Autodesk Inventor part; units mm, degrees
ref_plane "Work Plane1" through (-20, 3, 0) normal (0, -1, 0) x (1, 0, 0)
ref_plane "YZ Plane" through (0, 0, 0) normal (1, 0, 0) x (0, 1, 0)
ref_plane "XZ Plane" through (0, 0, 0) normal (0, 1, 0) x (-1, 0, 0)
sketch "Sketch1" plane through (0, 0, 0) normal (0, 0, 1) x (1, 0, 0)
  line L0 (0, 0) -> (0, -20)
  line L1 (0, 0) -> (-20, 0)
  line L2 (-20, 6) -> (0, 6)
  line L3 (6, 26) -> (6, -20)
  line L4 (-20, 0) -> (-20, 6)
  line L5 (0, -20) -> (6, -20)
  line L6 (0, 6) -> (0, 26)
  line L7 (0, 26) -> (6, 26)
  dimension "d0" = 20
  dimension "d1" = 20
  dimension "d2" = 6
  dimension "d3" = 26
  dimension "d4" = 6
  dimension "d5" = 46
extrude "Extrusion1" add sketch "Sketch1" along normal blind 20
sketch "Sketch2" plane through (-20, 0, 0) normal (0, -1, 0) x (1, 0, 0)
  line L0 (0, 20) -> (20, 20)
  line L1 (7, 20) -> (7, 0)
  line L2 (7, 0) -> (13, 0)
  line L3 (0, 0) -> (20, 0)
  line L4 (13, 0) -> (13, 20)
  line L5 (13, 20) -> (7, 20)
  line L6 (0, 0) -> (0, 20)
  dimension "d8" = 6
  dimension "d9" = 7
extrude "Extrusion2" add sketch "Sketch2" along normal blind 1.5 contours L0 L4 L2 L1
ref_plane "Work Plane1" through (-20, 3, 0) normal (0, -1, 0) x (1, 0, 0)
mirror "Mirror1" about plane through (-20, 3, 0) normal (0, -1, 0) of "Extrusion2"
sketch "Sketch3" plane through (6, -20, 0) normal (1, 0, 0) x (0, 0, -1)
  line L0 (0, 0) -> (-20, 0)
  line L1 (0, 0) -> (0, 46)
  line L2 (-20, 0) -> (-20, 46)
  line L3 (-20, 23) -> (0, 23)
  point P0 (0, 20)
  point P1 (-10, 10)
  point P2 (-10, 36)
  dimension "d13" = 10
  dimension "d14" = 10
hole "Hole1" at (6, -10, 10) at (6, 16, 10) direction (-1, 0, 0) diameter 5.5 end through all
sketch "Sketch4" plane through (6, -20, 0) normal (1, 0, 0) x (0, 0, -1)
  line L0 (-20, 20) -> (-20, 0)
  line L1 (-20, 10) -> (0, 10)
  line L2 (0, 20) -> (0, 0)
  line L3 (0, 0) -> (-20, 0)
  line L4 (-10, 0) -> (-10, 29.1489)
  line L5 (-20, 0) -> (-20, 46)
  line L6 (-20, 23) -> (0, 23)
  line L7 (0, 26) -> (0, 20)
  point P0 (-16, 4)
  point P1 (-16, 16)
  point P2 (-4, 4)
  point P3 (-4, 16)
  point P4 (-16, 42)
  point P5 (-16, 30)
  point P6 (-4, 42)
  point P7 (-4, 30)
  dimension "d22" = 6
  dimension "d23" = 6
hole "Hole2" at (6, -16, 16) at (6, -4, 16) at (6, -16, 4) at (6, -4, 4) at (6, 22, 16) at (6, 10, 16) at (6, 10, 4) at (6, 22, 4) direction (-1, 0, 0) diameter 3 end through all
fillet "Fillet1" radius 2 6 edges at (3, -20, 20) (3, 26, 20) (3, 26, 0) (3, -20, 0) (-20, 3, 20) (-20, 3, 0)
properties part number "Estrutura - Cabos"
For this review, take the finished solid that the model builds, in its own axes (mm). A direction names the side the tool comes from. Coordinates: 2 decimals unless noted, no trailing zeros. Loops run counter-clockwise (first coordinate to the right, second up) from the corner with the lowest first, then second, coordinate; pieces in that order, holes last. Notation, with made-up numbers: (-40, -19) -> (-33, -19) arc R21 ccw to (-33, -9) -> close; hole circle Ø9 at (-28.75, 13.25). An arc over 180 degrees is marked (long way). Write each question's results on one line, items separated by ' | '.
Q1. Add section D-D, the plane z = 6.5. State the section outline as (x, y) points.
Taken from the geometry:
outline: (-20, 0) -> (-13, 0) -> (-13, -1.5) -> (-7, -1.5) -> (-7, 0) -> (0, 0) -> (0, -20) -> (6, -20) -> (6, 26) -> (0, 26) -> (0, 6) -> (-7, 6) -> (-7, 7.5) -> (-13, 7.5) -> (-13, 6) -> (-20, 6) -> close
Q2. Add section A-A, the plane z = 4. Count the separate pieces of the cut face and the enclosed holes in it, then the cut area to 3 significant figures.
Taken from the geometry:
separate pieces: 5 | enclosed holes: 0 | area: 342 mm²
Q3. To check wall thickness, follow line 1 along Y through (x, z) = (3.65, 10); line 2 along Z through (x, y) = (2.2, 22); line 3 along Y through (x, z) = (3.8, 4). State the ranges of each line that lie inside material, in increasing order. Write a range as [from, to].
Taken from the geometry:
line 1: [-20, -12.75], [-7.25, 13.25], [18.75, 26] | line 2: [0, 2.5], [5.5, 14.5], [17.5, 20] | line 3: [-20, -17.5], [-14.5, -5.5], [-2.5, 8.5], [11.5, 20.5], [23.5, 26]
Q4. Add section C-C, the plane y = 16. State the section outline as (x, z) points.
Taken from the geometry:
outline: (0, 0) -> (6, 0) -> (6, 7.25) -> (0, 7.25) -> close; (0, 12.75) -> (6, 12.75) -> (6, 20) -> (0, 20) -> close
Q5. Machinability: for faces 1 (the flat face through (0, -12.1, 7.6)), 2 (the cylindrical face through (-19.43, 3.04, 19.4)), 3 (the flat face through (-10, 7.5, 10)), which of the approach directions +Z, -Z, +X, -X, +Y, -Y give a long, thin tool a straight path to every point of the face, cutting with its end or side? Answer none if there is none.
Taken from the geometry:
face 1: +Z, -Z, -Y | face 2: +Z, -X, +Y, -Y | face 3: +Z, -Z, -X, +Y
Q6. Add section B-B, the plane y = 10. State the section outline as (x, z) points, then the cut area to 3 significant figures.
Taken from the geometry:
outline: (0, 0) -> (6, 0) -> (6, 2.5) -> (0, 2.5) -> close; (0, 5.5) -> (6, 5.5) -> (6, 14.5) -> (0, 14.5) -> close; (0, 17.5) -> (6, 17.5) -> (6, 20) -> (0, 20) -> close | area: 84.0 mm²
Q7. Mouldability with a two-part tool opening along Z and no side actions: class faces 4 (the cylindrical face through (3.04, -19.43, 0.6)), 5 (the flat face through (-13, 7, 10)), 6 (the cylindrical face through (2.96, 20.99, 17.11)) as +Z half, -Z half, draft (parallel to the pull), parting line (faces both ways), or undercut.
Taken from the geometry:
face 4: -Z half | face 5: draft | face 6: undercut
Q8. For pin 1 Ø3.5 at (y, z) = (22, 16) entering from -X; pin 2 Ø2 at (x, z) = (-2.5, 14) entering from +Y; pin 3 Ø5.5 at (x, z) = (-15, 13.5) entering from +Y; pin 4 Ø5 at (y, z) = (-10, 10) entering from -X, all flat-tipped, find the tip position at first contact; note any pin that passes through.
Taken from the geometry:
pin 1: x = 0 | pin 2: y = 6 | pin 3: y = 7.5 | pin 4: through
